```python
from build123d import *

# Parameters (mm, degrees)
SKETCH1_W             = 609.6
SKETCH1_H             = 304.8
BOSS_EXTRUDE1_DEPTH   = 76.2
SKETCH2_W             = 533.4
SKETCH2_H             = 25.4
BOSS_EXTRUDE2_DEPTH   = 76.2
CUT_EXTRUDE1_DEPTH    = 688.678907631
SKETCH4_W             = 25.4
SKETCH4_H             = 76.2
BOSS_EXTRUDE3_DEPTH   = 76.2
SKETCH5_R             = 19.05
BOSS_EXTRUDE4_DEPTH   = 50.8
SKETCH6_R             = 25.4
BOSS_EXTRUDE7_DEPTH   = 6.35
FILLET1_R             = 12.7
MIRROR1_START         = -304.8
MIRROR1_DEPTH         = 25.4
MIRROR1_START_2       = -279.4
MIRROR1_2_OUTLINE_R   = 19.05
MIRROR1_2_DEPTH       = 57.15
MIRROR1_START_3       = -228.6
MIRROR1_3_OUTLINE_R   = 25.4
MIRROR1_3_OUTLINE_R_2 = 19.05
MIRROR1_3_DEPTH       = 6.35


# Read off the part's stored shape, not the designer's step: Mirror1
with BuildPart() as part:
    # Sketch1 → Boss-Extrude1 (new body)
    with BuildSketch(Plane(origin=(0, 0, 0), x_dir=(1, 0, 0), z_dir=(0, 1, 0))):
        with Locations((304.8, 152.4)):
            Rectangle(SKETCH1_W, SKETCH1_H)
    extrude(amount=BOSS_EXTRUDE1_DEPTH)

    # Sketch2 → Boss-Extrude2 (add)
    with BuildSketch(Plane(origin=(0, 76.2, 0), x_dir=(1, 0, 0), z_dir=(0, 1, 0))):
        with Locations((266.7, 12.7)):
            Rectangle(SKETCH2_W, SKETCH2_H)
    extrude(amount=BOSS_EXTRUDE2_DEPTH)

    # Sketch3 → Cut-Extrude1 (cut, through all)
    with BuildSketch(Plane(origin=(0, 0, -25.4), x_dir=(-1, 0, 0), z_dir=(0, 0, -1))):
        with BuildLine():
            Line((-508, 133.35), (-25.4, 133.35))
            ThreePointArc((-25.4, 133.35), (-6.35, 114.3), (-25.4, 95.25))
            Line((-25.4, 95.25), (-508, 95.25))
            ThreePointArc((-508, 95.25), (-527.05, 114.3), (-508, 133.35))
        make_face()
    extrude(amount=-CUT_EXTRUDE1_DEPTH, mode=Mode.SUBTRACT)

    # Sketch4 → Boss-Extrude3 (add, through all)
    with BuildSketch(Plane(origin=(533.4, 0, 0), x_dir=(0, 0, -1), z_dir=(1, 0, 0))):
        with Locations((12.7, 114.3)):
            Rectangle(SKETCH4_W, SKETCH4_H)
    extrude(amount=BOSS_EXTRUDE3_DEPTH)

    # Sketch5 → Boss-Extrude4 (add)
    with BuildSketch(Plane.XY.offset(-25.4)):
        with Locations((584.2, 114.3)):
            Circle(SKETCH5_R)
    extrude(amount=-BOSS_EXTRUDE4_DEPTH)

    # Sketch6 → Boss-Extrude7 (add)
    with BuildSketch(Plane(origin=(0, 0, -76.2), x_dir=(-1, 0, 0), z_dir=(0, 0, -1))):
        with Locations((-584.2, 114.3)):
            Circle(SKETCH6_R)
    extrude(amount=BOSS_EXTRUDE7_DEPTH)

    # Fillet1
    fillet1_edges = [part.edges().sort_by_distance(p)[0] for p in [
        (0, 152.4, -12.7),
        (609.6, 152.4, -12.7),
    ]]
    fillet(fillet1_edges, radius=FILLET1_R)

    # Mirror1 outline → Mirror1 (add)
    with BuildSketch(Plane.XY.offset(MIRROR1_START)):
        with BuildLine():
            Line((596.9, 152.4), (12.7, 152.4))
            ThreePointArc((12.7, 152.4), (3.719743879, 148.680256121), (0, 139.7))
            Line((0, 139.7), (0, 76.2))
            Line((0, 76.2), (609.6, 76.2))
            Line((609.6, 76.2), (609.6, 139.7))
            ThreePointArc((609.6, 139.7), (605.880256121, 148.680256121), (596.9, 152.4))
        make_face()
        with BuildLine():
            ThreePointArc((508, 133.35), (527.05, 114.3), (508, 95.25))
            Line((508, 95.25), (25.4, 95.25))
            ThreePointArc((25.4, 95.25), (6.35, 114.3), (25.4, 133.35))
            Line((25.4, 133.35), (508, 133.35))
        make_face(mode=Mode.SUBTRACT)
    extrude(amount=MIRROR1_DEPTH)

    # Mirror1 2 outline → Mirror1 2 (add)
    with BuildSketch(Plane.XY.offset(MIRROR1_START_2)):
        with Locations((584.2, 114.3)):
            Circle(MIRROR1_2_OUTLINE_R)
    extrude(amount=MIRROR1_2_DEPTH)

    # Mirror1 3 outline → Mirror1 3 (add)
    with BuildSketch(Plane.XY.offset(MIRROR1_START_3)):
        with Locations((584.2, 114.3)):
            Circle(MIRROR1_3_OUTLINE_R)
        with Locations((584.2, 114.3)):
            Circle(MIRROR1_3_OUTLINE_R_2, mode=Mode.SUBTRACT)
    extrude(amount=MIRROR1_3_DEPTH)


solid = part.part
```
Work out the finished part from the listing and answer in its coordinate system (mm). A direction names the side the tool comes from. Give positions to 0.01 mm unless a question says otherwise; leave off trailing zeros. Order: outer loops, then holes, each group sorted by start corner. A loop starts at its lowest first (then second) coordinate and runs counter-clockwise, first axis right, second up. Notation, with made-up numbers: (41, -34.75) - (83, -34.75) arc R19 ccw to (83, -12.75) - close; hole circle Ø4 at (82.25, 54). An arc over 180 degrees is marked (long way). One line per item, written item: value. Start each with the question number.
1. Each of these flat-tipped pins is pushed along its axis until it touches: pin 1 Ø1 at (y, z) = (109.5, -267) entering from -X; pin 2 Ø5 at (x, z) = (161, -241) entering from +Y. Where does it stop, or does it pass through?
2. Section B-B, the plane x = 165 is taken. Write down the section's boundary in (y, z), then the cut area to 3 significant figures.
3. Section D-D, the plane x = 584.2 is taken. Write down the section's boundary in (y, z), then the cut area to 3 significant figures.
4. Section A-A, the plane y = 114.3 is taken. Count the separate pieces of the cut face and the enclosed holes in it, then the cut area to 3 significant figures.
5. Which of the six approach directions +Z, -Z, +X, -X, +Y, -Y give full straight-line access (tool end or side, diameter ignored) to faces 1 (the face through (263, 95.25, -13)), 2 (the face through (601.797, 107.004, -254.356)), 3 (the face through (584, 115, -222.25))?
6. Consider line 1 (Y direction, x = 489, z = -14); line 2 (Z direction, x = 546, y = 84); line 3 (Y direction, x = 125, z = -169.5). Determine where each line is inside the solid, lowest interval first.
7. Section C-C, the plane z = -45.5 is taken. Write down the section's boundary in (x, y), then the cut area to 3 significant figures.
8. For a pull along Z with two mould halves and no side action, classify faces 4 (the face through (604.357, 98.844, -79.331)), 5 (the face through (301, 58, 0)), 6 (the face through (301, 152.4, -13)) as released by +Z, released by -Z, zero draft, split by the parting line, or undercut.
Filled sheet:
1. pin 1: x = 565.64
1. pin 2: y = 76.2
2. outline: (0, -304.8) - (95.25, -304.8) - (95.25, -279.4) - (76.2, -279.4) - (76.2, -25.4) - (95.25, -25.4) - (95.25, 0) - (0, 0) - close; (133.35, -304.8) - (152.4, -304.8) - (152.4, -279.4) - (133.35, -279.4) - close; (133.35, -25.4) - (152.4, -25.4) - (152.4, 0) - (133.35, 0) - close
2. area: 25,200 mm²
3. outline: (0, -304.8) - (152.4, -304.8) - (152.4, -279.4) - (133.35, -279.4) - (133.35, -228.6) - (139.7, -228.6) - (139.7, -222.25) - (88.9, -222.25) - (88.9, -228.6) - (95.25, -228.6) - (95.25, -279.4) - (76.2, -279.4) - (76.2, -25.4) - (95.25, -25.4) - (95.25, -76.2) - (88.9, -76.2) - (88.9, -82.55) - (139.7, -82.55) - (139.7, -76.2) - (133.35, -76.2) - (133.35, -25.4) - (152.4, -25.4) - (152.4, 0) - (0, 0) - close
3. area: 31,600 mm²
4. separate pieces: 4
4. enclosed holes: 0
4. area: 9,030 mm²
5. face 1: +Z, -Z
5. face 2: none
5. face 3: +X, -X, +Y
6. line 1: 0 to 95.25, 133.35 to 152.4
6. line 2: -304.8 to -279.4, -25.4 to 0
6. line 3: 0 to 76.2
7. outline: (0, 0) - (609.6, 0) - (609.6, 76.2) - (0, 76.2) - close; circle Ø38.1 at (584.2, 114.3)
7. area: 47,600 mm²
8. face 4: undercut
8. face 5: released by +Z
8. face 6: zero draft
